Check sheet for the modelled part. Datum: model origin and axes. Units: mm. Face numbers are marked on the shaded views. A direction names the side the tool comes from. Round coordinates to 2 decimals unless told otherwise and drop trailing zeros. Order: outer loops, then holes, each group sorted by start corner. A loop starts at its lowest first (then second) coordinate and runs counter-clockwise, first axis right, second up.
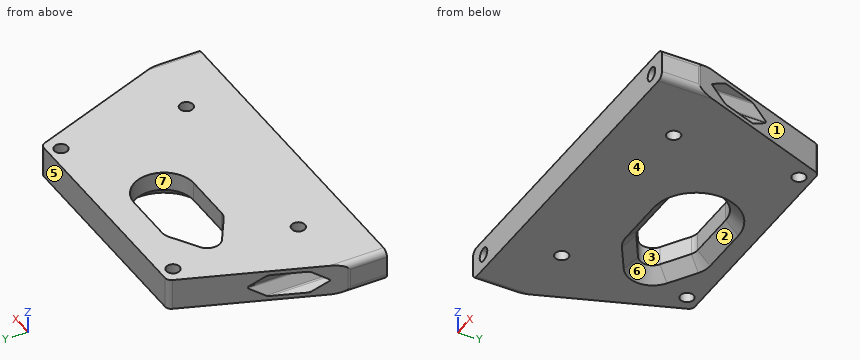
```python
from build123d import *

# Parameters (mm, degrees)
SKETCH_1_R          = 2.15
EXTRUDE_1_DEPTH     = 10
SKETCH_2_R          = 2.15
CUT_EXTRUDE_1_DEPTH = 82.338797631
CUT_EXTRUDE_2_DEPTH = 50
FILLET_1_R          = 0.5
FILLET_2_R          = 2
SKETCH_4_R          = 9.478521267
SKETCH_4_R_2        = 4.478521267
SKETCH_4_R_3        = 4.1275
CUT_EXTRUDE_3_DEPTH = 82.338797631
CHAMFER_1_SIZE      = 4


with BuildPart() as part:
    # 草图1 → 凸台-拉伸1 (new body)
    with BuildSketch(Plane.XY):
        Polygon((-54, 0), (54, 0), (54, 12), (36, 60), (-36, 60), (-54, 12), align=None)
        with Locations((-32, 56)):
            Circle(SKETCH_1_R, mode=Mode.SUBTRACT)
        with Locations((32, 56)):
            Circle(SKETCH_1_R, mode=Mode.SUBTRACT)
        with Locations((32, 16)):
            Circle(SKETCH_1_R, mode=Mode.SUBTRACT)
        with Locations((-32, 16)):
            Circle(SKETCH_1_R, mode=Mode.SUBTRACT)
    extrude(amount=EXTRUDE_1_DEPTH)

    # 草图2 → 切除-拉伸1 (cut, through all)
    with BuildSketch(Plane.XZ):
        with Locations(Location((48, 5, 0), (0, 0, 270))):
            Circle(SKETCH_2_R)
        with Locations(Location((-48, 5, 0), (0, 0, 180))):
            Circle(SKETCH_2_R)
    extrude(amount=-CUT_EXTRUDE_1_DEPTH, mode=Mode.SUBTRACT)

    # 草图3 → 切除-拉伸2 (cut)
    with BuildSketch(Plane(origin=(0, 60, 0), x_dir=(1, 0, 0), z_dir=(0, 1, 0))):
        Polygon((-43.814210548, -5), (-45.907105274, -1.375), (-50.092894726, -1.375), (-52.185789452, -5), (-50.092894726, -8.625), (-45.907105274, -8.625), align=None)
        Polygon((43.814210548, -5), (45.907105274, -8.625), (50.092894726, -8.625), (52.185789452, -5), (50.092894726, -1.375), (45.907105274, -1.375), align=None)
    extrude(amount=-CUT_EXTRUDE_2_DEPTH, mode=Mode.SUBTRACT)

    # 圆角1
    fillet_1_edges = [part.edges().sort_by_distance(p)[0] for p in [
        (-43.814210548, 24.581052602, 5),
        (-45.907105274, 21.790526301, 8.625),
        (-50.092894726, 16.209473699, 8.625),
        (-52.185789452, 13.418947398, 5),
        (-50.092894726, 16.209473699, 1.375),
        (-45.907105274, 21.790526301, 1.375),
        (43.814210548, 24.581052602, 5),
        (45.907105274, 21.790526301, 1.375),
        (50.092894726, 16.209473699, 1.375),
        (52.185789452, 13.418947398, 5),
        (50.092894726, 16.209473699, 8.625),
        (45.907105274, 21.790526301, 8.625),
    ]]
    fillet(fillet_1_edges, radius=FILLET_1_R)

    # 圆角2
    fillet_2_edges = [part.edges().sort_by_distance(p)[0] for p in [
        (-54, 12, 5),
        (-36, 60, 5),
        (36, 60, 5),
        (54, 12, 5),
        (-54, 6, 10),
        (54, 6, 10),
        (-54, 6, 0),
        (54, 6, 0),
    ]]
    fillet(fillet_2_edges, radius=FILLET_2_R)

    # 草图4 → 切除-拉伸3 (cut, through all)
    with BuildSketch(Plane(origin=(0, 0, 0), x_dir=(-1, 0, 0), z_dir=(0, 0, -1))):
        with Locations((0, 41)):
            Circle(SKETCH_4_R)
        with BuildLine():
            Line((26.84820546, 44.499874972), (18.374024707, 49.797520169))
            ThreePointArc((18.374024707, 49.797520169), (19.917223052, 48.170833089), (20.478521267, 46))
            ThreePointArc((20.478521267, 46), (12.833207242, 42.833207242), (16, 50.478521267))
            Line((16, 50.478521267), (0, 50.478521267))
            ThreePointArc((0, 50.478521267), (6.702326663, 47.702326663), (9.478521267, 41))
            ThreePointArc((9.478521267, 41), (6.702326663, 34.297673337), (0, 31.521478733))
            Line((0, 31.521478733), (16, 31.521478733))
            ThreePointArc((16, 31.521478733), (12.833207242, 39.166792758), (20.478521267, 36))
            ThreePointArc((20.478521267, 36), (19.917223052, 33.829166911), (18.374024707, 32.202479831))
            Line((18.374024707, 32.202479831), (26.84820546, 37.500125028))
            ThreePointArc((26.84820546, 37.500125028), (20.532754038, 41), (26.84820546, 44.499874972))
        make_face()
        with Locations((16, 46)):
            Circle(SKETCH_4_R_2)
        with Locations((16, 36)):
            Circle(SKETCH_4_R_2)
        with Locations((24.660254038, 41)):
            Circle(SKETCH_4_R_3)
    extrude(amount=-CUT_EXTRUDE_3_DEPTH, mode=Mode.SUBTRACT)

    # 倒角1
    chamfer_1_edges = [part.edges().sort_by_distance(p)[0] for p in [
        (-8, 50.478521267, 0),
        (-22.611115084, 47.14869757, 0),
        (9.478521267, 41, 0),
        (-8, 31.521478733, 0),
        (-17.234884185, 31.695094218, 0),
        (-22.611115084, 34.85130243, 0),
        (-28.787754038, 41, 0),
        (-17.234884185, 50.304905782, 0),
    ]]
    chamfer(chamfer_1_edges, length=CHAMFER_1_SIZE)


solid = part.part
```
Item 1: Scan lines: line 1 along X through (y, z) = (6.5, 5); line 2 along Y through (x, z) = (-32, 7.5); line 3 along Y through (x, z) = (-14, 8). Record each from-to range of solid material in increasing order.
Answer:
line 1: x = -54 to -50.15, -45.85 to 45.85, 50.15 to 54
line 2: y = 0 to 13.85, 18.15 to 53.85, 58.15 to 60
line 3: y = 0 to 31.52, 50.48 to 60
Item 2: Sectioned sample at C-C (y = 15). State how many separate pieces and enclosed holes the cut face has, and give its area (3 significant figures).
Answer:
separate pieces: 3
enclosed holes: 2
area: 890 mm2
Item 3: Sectioned sample at A-A (x = -48). Record the cut outline in (y, z) (3 decimals), and give its area (4 significant figures).
Answer:
outline: (0, 0) - (28, 0) - (28, 1.375) - (10, 1.375) - (10, 2.85) - (0, 2.85) - close; (0, 7.15) - (10, 7.15) - (10, 8.625) - (28, 8.625) - (28, 10) - (0, 10) - close
area: 106.5 mm2
Item 4: Access from +Z, -Z, +X, -X, +Y, -Y to the whole of each face (thin tool, end or side, straight path). Record for the marked faces 5, 6 and 7.
Answer:
face 5: +Z, -Z, +X, -X, +Y
face 6: -Z
face 7: +Z, -Z
Item 5: Go/stop test with flat-tipped pins: P1, Ø1, axis at x = 32.5, z = 8, coming from the -Y side; P2, Ø3.5, axis at x = -48, z = 4, coming from the +Y side; P3, Ø2, axis at y = 26, z = 2, coming from the -X side. Record where each tip stops, or that it passes through.
Answer:
P1: stops at y = 0
P2: stops at y = 10
P3: stops at x = -49.04
Item 6: Sectioned sample at B-B (x = 32). Record the cut outline in (y, z), and give its area (3 significant figures).
Answer:
outline: (0, 0) - (13.85, 0) - (13.85, 10) - (0, 10) - close; (18.15, 0) - (53.85, 0) - (53.85, 10) - (18.15, 10) - close; (58.15, 0) - (60, 0) - (60, 10) - (58.15, 10) - close
area: 514 mm2
Item 7: Release check for a two-part mould opening along X. For the marked faces 1, 2, 3 and 4 record: released by +X, released by -X, zero draft, split by the parting line, or undercut.
Answer:
face 1: released by +X
face 2: undercut
face 3: undercut
face 4: zero draft
